```python
from build123d import *

# Parameters (mm, degrees)
F0_R     = 50
F1_DEPTH = 14.9
F2_R     = 50
F2_R_2   = 25
F3_DEPTH = 105
F4_W     = 30
F4_H     = 30
F5_DEPTH = 0.1


with BuildPart() as f1:
    # F0 (on Top) → F1 (new body)
    with BuildSketch(Plane.XY):
        Circle(F0_R)
    extrude(amount=F1_DEPTH)

    # F2 (on face) → F3 (join)
    with BuildSketch(Plane.XY.offset(14.9)):
        Circle(F2_R)
        Circle(F2_R_2, mode=Mode.SUBTRACT)
    extrude(amount=F3_DEPTH)

    # F4 (on face) → F5 (join)
    with BuildSketch(Plane(origin=(0, 0, 0), x_dir=(1, 0, 0), z_dir=(0, 0, -1))):
        Rectangle(F4_W, F4_H)
    extrude(amount=F5_DEPTH)


solid = f1.part
```
Geometry check sheet. Reference: the model listing, model coordinates, mm. A direction names the side the tool comes from. Round coordinates to 2 decimals unless told otherwise and drop trailing zeros. Order: outer loops, then holes, each group sorted by start corner. A loop starts at its lowest first (then second) coordinate and runs counter-clockwise, first axis right, second up. Notation, with made-up numbers: (54.5, 71) -> (102.5, 71) arc R14 ccw to (102.5, 93) -> close; hole circle Ø2 at (61, 62). An arc over 180 degrees is marked (long way). Return JSON: item names as keys, results as strings. Group by question number.
Q1. Section check A-A, the plane y = 0. Record the boundary of the cut face in (x, z).
Q2. Section check C-C, the plane z = 62. Record the boundary of the cut face in (x, y), plus the area to 3 significant figures.
Q3. Gauge pin test, flat ends, axial feed: pin 1 (1 mm diameter, centred on x = -13, z = 38.5, fed in from -Y); pin 2 (1.5 mm diameter, centred on x = 7.5, z = 89, fed in from +Y); pin 3 (4 mm diameter, centred on x = -20, y = -15.5, fed in from -Z). Record the tip position at first contact, or that the pin passes through.
Q4. Material ranges on probe 1 along Y at (x, z) = (0, 93); probe 2 along Z at (x, y) = (31.5, -13.5); probe 3 along Z at (x, y) = (7, -19.5), recorded low to high. Write a range as from..to.
Q5. Tool access check on faces 1 (the flat face through (-22.9, -10.4, 119.9)), 2 (the flat face through (0, 0, 14.9)). Record the directions out of +Z, -Z, +X, -X, +Y, -Y that give a thin tool (end or side, any length) a straight path to the whole face; none if there is none.
Q6. Section check D-D, the plane z = 10. Record the boundary of the cut face in (x, y), plus the area to 3 significant figures.
Q7. Release check for a two-part mould opening along X. For faces 3 (the cylindrical face through (47.69, 15.02, 59.11)), 4 (the flat face through (-1, -22, 0)), 5 (the cylindrical face through (23.846, 7.509, 66.665)) record: released by +X, released by -X, zero draft, split by the parting line, or undercut.
Numbers:
{
 "1": {"outline": "(-50, 0) -> (-15, 0) -> (-15, -0.1) -> (15, -0.1) -> (15, 0) -> (50, 0) -> (50, 119.9) -> (25, 119.9) -> (25, 14.9) -> (-25, 14.9) -> (-25, 119.9) -> (-50, 119.9) -> close"},
 "2": {"outline": "circle Ø100 at (0, 0); hole circle Ø50 at (0, 0)", "area": "5,890 mm^2"},
 "3": {"pin 1": "y = -48.41", "pin 2": "y = 49.54", "pin 3": "z = 0"},
 "4": {"probe 1": "-50..-25, 25..50", "probe 2": "0..119.9", "probe 3": "0..14.9"},
 "5": {"face 1": "+Z, +X, -X, +Y, -Y", "face 2": "+Z"},
 "6": {"outline": "circle Ø100 at (0, 0)", "area": "7,850 mm^2"},
 "7": {"face 3": "split by the parting line", "face 4": "zero draft", "face 5": "undercut"}
}
